Geometry check sheet. Reference: the model listing, model coordinates, mm. Face numbers are marked on the shaded views. A direction names the side the tool comes from. Round coordinates to 2 decimals unless told otherwise and drop trailing zeros. Write each loop counter-clockwise with the first axis right and the second up, starting at its lowest first coordinate (ties: lowest second). Pieces come first, ordered by that corner, then holes. Notation, with made-up numbers: (14.5, 6) -> (30.5, 6) arc R25 ccw to (30.5, 44) -> close; hole circle Ø3 at (63, 84). An arc over 180 degrees is marked (long way). Use a Markdown table: item, result.
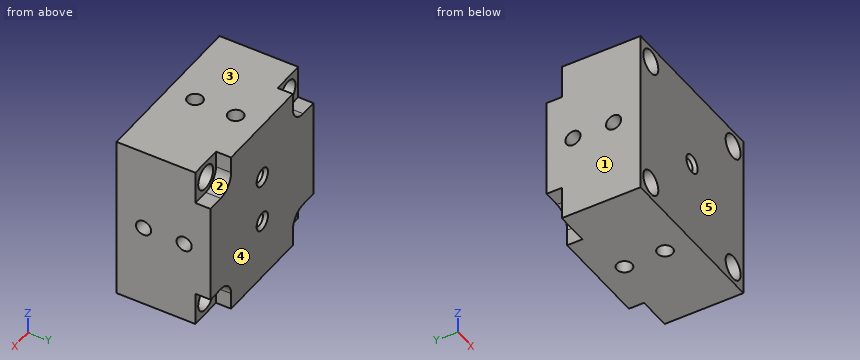
```python
from build123d import *

# Parameters (mm, degrees)
SKETCH_1_W                   = 55
SKETCH_1_H                   = 55
EXTRUDE_1_DEPTH              = 15.5
CUT_EXTRUDE_1_DEPTH          = 5
SKETCH_4_R                   = 4
CUT_EXTRUDE_2_DEPTH          = 47.781406563
PATTERN_LINEAR_3_COUNT       = 2
PATTERN_LINEAR_3_PITCH       = 16
PATTERN_LINEAR_4_COUNT       = 2
PATTERN_LINEAR_4_PITCH       = 13.4
PATTERN_CIRCULAR_2_COUNT     = 4
HOLE_WIZARD_M6_3_D           = 4
HOLE_WIZARD_M6_3_DEPTH       = 7
HOLE_WIZARD_M6_3_CSINK_D     = 6.05
HOLE_WIZARD_M6_3_CSINK_ANGLE = 90
HOLE_WIZARD_M6_3_TIP         = 1.201721238


with BuildPart() as part:
    # 草图1 → 凸台-拉伸1 (new, symmetric)
    with BuildSketch(Plane(origin=(0, 0, 0), x_dir=(1, 0, 0), z_dir=(0, 1, 0))):
        Rectangle(SKETCH_1_W, SKETCH_1_H)
    extrude(amount=EXTRUDE_1_DEPTH, both=True)

    # 草图2 → 切除-拉伸1 (cut)
    with BuildSketch(Plane(origin=(0, 15.5, 0), x_dir=(1, 0, 0), z_dir=(0, 1, 0))):
        with BuildLine():
            Line((16.5, 22), (16.5, 27.5))
            Line((16.5, 27.5), (27.5, 27.5))
            Line((27.5, 27.5), (27.5, 16.5))
            Line((27.5, 16.5), (21.999999502, 16.5))
            ThreePointArc((21.999999502, 16.5), (18.110912527, 18.11091288), (16.5, 22))
        make_face()
        with BuildLine():
            Line((22, -16.5), (27.5, -16.5))
            Line((27.5, -16.5), (27.5, -27.5))
            Line((27.5, -27.5), (16.5, -27.5))
            Line((16.5, -27.5), (16.5, -21.999999502))
            ThreePointArc((16.5, -21.999999502), (18.11091288, -18.110912527), (22, -16.5))
        make_face()
        with BuildLine():
            Line((-16.5, -22), (-16.5, -27.5))
            Line((-16.5, -27.5), (-27.5, -27.5))
            Line((-27.5, -27.5), (-27.5, -16.5))
            Line((-27.5, -16.5), (-21.999999502, -16.5))
            ThreePointArc((-21.999999502, -16.5), (-18.110912527, -18.11091288), (-16.5, -22))
        make_face()
        with BuildLine():
            Line((-22, 16.5), (-27.5, 16.5))
            Line((-27.5, 16.5), (-27.5, 27.5))
            Line((-27.5, 27.5), (-16.5, 27.5))
            Line((-16.5, 27.5), (-16.5, 21.999999502))
            ThreePointArc((-16.5, 21.999999502), (-18.11091288, 18.110912527), (-22, 16.5))
        make_face()
    extrude(amount=-CUT_EXTRUDE_1_DEPTH, mode=Mode.SUBTRACT)

    # 草图4 → 切除-拉伸2 (cut, through all)
    with BuildSketch(Plane(origin=(0, 10.5, 0), x_dir=(1, 0, 0), z_dir=(0, 1, 0))):
        with Locations(Location((22, 22, 0), (0, 0, 270))):
            Circle(SKETCH_4_R)
        with Locations(Location((22, -22, 0), (0, 0, 270))):
            Circle(SKETCH_4_R)
        with Locations(Location((-22, -22, 0), (0, 0, 270))):
            Circle(SKETCH_4_R)
        with Locations(Location((-22, 22, 0), (0, 0, 270))):
            Circle(SKETCH_4_R)
    extrude(amount=-CUT_EXTRUDE_2_DEPTH, mode=Mode.SUBTRACT)

    # 草图6 → M6 螺纹孔1 (revolve, cut)
    with BuildSketch(Plane(origin=(-0.027335572, -6.601540671, 27.5), x_dir=(0, -1, 0), z_dir=(1, 0, 0))):
        Polygon((0, 0), (0, 8.502151548), (2.5, 7), (2.5, -0.5), (2, 0), align=None)
    hole_wizard_m6_1 = revolve(axis=Axis((-0.027335572, -6.601540671, 33.85), (0, 0, -1)), mode=Mode.SUBTRACT)

    # 草图8 → M6 螺纹孔2 (revolve, cut)
    with BuildSketch(Plane(origin=(-0.182583925, 15.5, -7.358132173), x_dir=(0, 0, 1), z_dir=(1, 0, 0))):
        Polygon((0, 0), (0, 8.201721238), (2, 7), (2, 1.025), (3.025, 0), align=None)
    hole_wizard_m6_2 = revolve(axis=Axis((-0.182583925, 21.85, -7.358132173), (0, -1, 0)), mode=Mode.SUBTRACT)

    # 阵列(线性)3: M6 螺纹孔2 ×2
    with Locations(*[(0, 0, i * PATTERN_LINEAR_3_PITCH) for i in range(1, PATTERN_LINEAR_3_COUNT)]):
        add(hole_wizard_m6_2, mode=Mode.SUBTRACT)

    # 阵列(线性)4: M6 螺纹孔1 ×2
    with Locations(*[(0, i * PATTERN_LINEAR_4_PITCH, 0) for i in range(1, PATTERN_LINEAR_4_COUNT)]):
        add(hole_wizard_m6_1, mode=Mode.SUBTRACT)

    # 阵列(圆周)2: M6 螺纹孔1 ×4 about axis
    pattern_circular_2_axis = Axis((0, 0, 0), (0, 1, 0))
    for i in range(1, PATTERN_CIRCULAR_2_COUNT):
        add(hole_wizard_m6_1.rotate(pattern_circular_2_axis, i * 360 / PATTERN_CIRCULAR_2_COUNT), mode=Mode.SUBTRACT)

    # 阵列(圆周)2 copy 1 sketch → 阵列(圆周)2 copy 1 (revolve, cut)
    with BuildSketch(Plane(origin=(27.5, 6.798459329, 0.027335572), x_dir=(0, -1, 0), z_dir=(0, 0, -1))):
        Polygon((0, 0), (0, 8.502151548), (2.5, 7), (2.5, -0.5), (2, 0), align=None)
    revolve(axis=Axis((33.85, 6.798459329, 0.027335572), (-1, 0, 0)), mode=Mode.SUBTRACT)

    # 阵列(圆周)2 copy 2 sketch → 阵列(圆周)2 copy 2 (revolve, cut)
    with BuildSketch(Plane(origin=(0.027335572, 6.798459329, -27.5), x_dir=(0, -1, 0), z_dir=(-1, 0, 0))):
        Polygon((0, 0), (0, 8.502151548), (2.5, 7), (2.5, -0.5), (2, 0), align=None)
    revolve(axis=Axis((0.027335572, 6.798459329, -33.85), (0, 0, 1)), mode=Mode.SUBTRACT)

    # 阵列(圆周)2 copy 3 sketch → 阵列(圆周)2 copy 3 (revolve, cut)
    with BuildSketch(Plane(origin=(-27.5, 6.798459329, -0.027335572), x_dir=(0, -1, 0), z_dir=(0, 0, 1))):
        Polygon((0, 0), (0, 8.502151548), (2.5, 7), (2.5, -0.5), (2, 0), align=None)
    revolve(axis=Axis((-33.85, 6.798459329, -0.027335572), (1, 0, 0)), mode=Mode.SUBTRACT)

    # M6 螺纹孔3
    with Locations(Plane(origin=(-6.578522575, -15.5, 8.386748618), x_dir=(-1, 0, 0), z_dir=(0, -1, 0))):
        with Locations((-6.578522575, 8.156808217)):
            CounterSinkHole(HOLE_WIZARD_M6_3_D / 2, HOLE_WIZARD_M6_3_CSINK_D / 2, depth=HOLE_WIZARD_M6_3_DEPTH, counter_sink_angle=HOLE_WIZARD_M6_3_CSINK_ANGLE)
            with Locations((0, 0, -(HOLE_WIZARD_M6_3_DEPTH + HOLE_WIZARD_M6_3_TIP / 2))):  # 118° drill point
                Cone(0, HOLE_WIZARD_M6_3_D / 2, HOLE_WIZARD_M6_3_TIP, mode=Mode.SUBTRACT)


solid = part.part
```
(1) Thickness scan on line 1 (Z direction, x = -24.5, y = 10); line 2 (X direction, y = -11, z = 21); line 3 (Z direction, x = -24, y = 6.5). Record the ranges inside material, lowest first.
A:
| item | result |
|---|---|
| line 1 | z = -27.5 to -25.12, -18.88 to 18.88, 25.12 to 27.5 |
| line 2 | x = -27.5 to -25.87, -18.13 to 18.13, 25.87 to 27.5 |
| line 3 | z = -27.5 to -25.46, -18.54 to -2.51, 2.45 to 18.54, 25.46 to 27.5 |
(2) Section check B-B on y = -10.5. Record the cut outline in (x, z), plus the area to 3 significant figures.
A:
| item | result |
|---|---|
| outline | (-27.5, -27.5) -> (27.5, -27.5) -> (27.5, 27.5) -> (-27.5, 27.5) -> close; hole circle Ø8 at (-22, -22); hole circle Ø8 at (-22, 22); hole circle Ø4 at (0, 0.23); hole circle Ø8 at (22, -22); hole circle Ø8 at (22, 22) |
| area | 2,810 mm2 |
(3) Gauge pin test, flat ends, axial feed: pin 1 Ø5.5 at (x, y) = (-24.5, 13) entering from -Z; pin 2 Ø1.5 at (x, y) = (25, 13) entering from +Z; pin 3 Ø3.5 at (x, z) = (20, -22.5) entering from +Y; pin 4 Ø2.5 at (y, z) = (13.5, 25) entering from +X. Record the tip position at first contact, or that the pin passes through.
A:
| item | result |
|---|---|
| pin 1 | stops at z = -27.5 |
| pin 2 | stops at z = 16.5 |
| pin 3 | passes through |
| pin 4 | stops at x = 16.5 |
(4) Section check A-A on y = -0.5. Record the cut outline in (x, z).
A:
| item | result |
|---|---|
| outline | (-27.5, -27.5) -> (27.5, -27.5) -> (27.5, 27.5) -> (-27.5, 27.5) -> close; hole circle Ø8 at (-22, -22); hole circle Ø8 at (-22, 22); hole circle Ø8 at (22, -22); hole circle Ø8 at (22, 22) |
(5) Access from +Z, -Z, +X, -X, +Y, -Y to the whole of each face (thin tool, end or side, straight path). Record for the marked faces 1 and 2.
A:
| item | result |
|---|---|
| face 1 | +Z, -Z, -X, +Y, -Y |
| face 2 | +Z, +X, +Y |
(6) Release check for a two-part mould opening along Y. For the marked faces 3, 4 and 5 record: +Y half, -Y half, draft (parallel to the pull), parting line (faces both ways), or undercut.
A:
| item | result |
|---|---|
| face 3 | draft |
| face 4 | +Y half |
| face 5 | -Y half |
